For this review, take the finished solid that the model builds, in its own axes (mm). A direction names the side the tool comes from. Give positions to 0.01 mm unless a question says otherwise; leave off trailing zeros. Write each loop counter-clockwise with the first axis right and the second up, starting at its lowest first coordinate (ties: lowest second). Pieces come first, ordered by that corner, then holes. Notation, with made-up numbers: (17.25, -11) -> (57.25, -11) arc R11 ccw to (57.25, 2) -> close; hole circle Ø11 at (85, 15). An arc over 180 degrees is marked (long way). Return JSON: item names as keys, results as strings.
Autodesk Inventor part; units mm, degrees
ref_plane "YZ Plane" through (0, 0, 0) normal (1, 0, 0) x (0, 1, 0)
ref_plane "XZ Plane" through (0, 0, 0) normal (0, 1, 0) x (-1, 0, 0)
ref_plane "XY Plane" through (0, 0, 0) normal (0, 0, 1) x (1, 0, 0)
sketch "Sketch1" plane through (0, 0, 0) normal (0, 0, 1) x (1, 0, 0)
  line L0 (0, 0) -> (92, 0)
  line L1 (92, 0) -> (92, 87.5)
  line L2 (0, 87.5) -> (0, 0)
  line L3 (0, 87.5) -> (4, 91.5)
  line L4 (92, 87.5) -> (88, 91.5)
  line L5 (4, 91.5) -> (4, 183.5)
  line L6 (88, 91.5) -> (88, 151.5)
  line L7 (34.5, 21) -> (57.5, 21)
  line L8 (58.5, 20) -> (58.5, 11)
  line L9 (57.5, 10) -> (34.5, 10)
  line L10 (33.5, 11) -> (33.5, 20)
  arc A0 (34.5, 21) -> (33.5, 20) centre (34.5, 20) ccw
  arc A1 (33.5, 11) -> (34.5, 10) centre (34.5, 11) ccw
  arc A2 (57.5, 10) -> (58.5, 11) centre (57.5, 11) ccw
  arc A3 (58.5, 20) -> (57.5, 21) centre (57.5, 20) ccw
  line L11 (9, 75) -> (32, 75)
  line L12 (33, 74) -> (33, 65)
  line L13 (32, 64) -> (9, 64)
  line L14 (8, 65) -> (8, 74)
  arc A4 (9, 75) -> (8, 74) centre (9, 74) ccw
  arc A5 (8, 65) -> (9, 64) centre (9, 65) ccw
  arc A6 (32, 64) -> (33, 65) centre (32, 65) ccw
  arc A7 (33, 74) -> (32, 75) centre (32, 74) ccw
  arc A8 (59, 65) -> (60, 64) centre (60, 65) ccw
  arc A9 (60, 75) -> (59, 74) centre (60, 74) ccw
  line L15 (83, 64) -> (60, 64)
  line L16 (84, 74) -> (84, 65)
  arc A10 (83, 64) -> (84, 65) centre (83, 65) ccw
  arc A11 (84, 74) -> (83, 75) centre (83, 74) ccw
  line L17 (60, 75) -> (83, 75)
  line L18 (59, 65) -> (59, 74)
  line L19 (4, 183.5) -> (36, 183.5)
  line L20 (36, 183.5) -> (36, 151.5)
  line L21 (36, 151.5) -> (88, 151.5)
  point P0 (46, 10)
  point P1 (46, 0)
  point P2 (84, 69.5)
  point P3 (58.5, 15.5)
  dimension "d0" = 92
  dimension "d1" = 135
  dimension "d2" = 1
  dimension "d3" = 11
  dimension "d4" = 25
  dimension "d5" = 1
  dimension "d6" = 11
  dimension "d7" = 25
  dimension "d8" = 1
  dimension "d9" = 11
  dimension "d10" = 25
  dimension "d11" = 4
  dimension "d12" = 54
  dimension "d13" = 8
  dimension "d14" = 8
  dimension "d15" = 10
  dimension "d16" = 32
  dimension "d17" = 32
  dimension "d18" = 183.5
  dimension "d19" = 87.5
extrude "Extrusion1" add sketch "Sketch1" along normal blind 6
sketch "Sketch2" plane through (0, 0, 6) normal (0, 0, 1) x (1, 0, 0)
  line L0 (34.5, 21) -> (57.5, 21)
  line L1 (33.5, 11) -> (33.5, 20)
  line L2 (34, 23) -> (58, 23) construction
  line L3 (58, 23) -> (58, 8) construction
  line L4 (58, 8) -> (34, 8) construction
  line L5 (34, 8) -> (34, 23) construction
  circle A0 centre (31.75, 32) radius 2.25
  circle A1 centre (60.25, 32) radius 2.25
  line L6 (31.75, 32) -> (60.25, 32) construction
  point P0 (34, 15.5)
  point P1 (33.5, 15.5)
  point P2 (46, 23)
  point P3 (46, 21)
  point P4 (46, 32)
  dimension "d22" = 24
  dimension "d23" = 15
  dimension "d24" = 4.5
  dimension "d25" = 28.5
  dimension "d26" = 9
extrude "Extrusion2" cut sketch "Sketch2" against normal blind 6
sketch "Sketch3" plane through (0, 0, 6) normal (0, 0, 1) x (1, 0, 0)
  circle A0 centre (31.75, 32) radius 2.25
  circle A1 centre (60.25, 32) radius 2.25
  line L0 (16.25, 35) -> (24.25, 35)
  line L1 (24.25, 35) -> (24.25, 29)
  line L2 (24.25, 29) -> (16.25, 29)
  line L3 (16.25, 29) -> (16.25, 35)
  line L4 (67.75, 35) -> (75.75, 35)
  line L5 (75.75, 35) -> (75.75, 29)
  line L6 (75.75, 29) -> (67.75, 29)
  line L7 (67.75, 29) -> (67.75, 35)
  point P0 (24.25, 32)
  dimension "d29" = 6
  dimension "d30" = 8
  dimension "d31" = 8
  dimension "d32" = 7.5
  dimension "d33" = 7.5
extrude "Extrusion3" cut sketch "Sketch3" against normal blind 6 contours L0 L1 L2 L3 | L4 L5 L6 L7
equation "\"d14\" = d13"
properties part number "x_carriage_front"
1. Add section D-D, the plane y = 157.5. State the section outline as (x, z) points, plus the area to 3 significant figures.
Results found:
{"outline": "(4, 0) -> (36, 0) -> (36, 6) -> (4, 6) -> close", "area": "192 mm²"}
2. The part is to be moulded in two halves that separate along X. For faces 1 (the flat face through (88, 121, 3)), 2 (the flat face through (62, 151.5, 3)), 3 (the flat face through (46, 10, 3)), say which applies: +X half, -X half, draft (parallel to the pull), parting line (faces both ways), or undercut.
Results found:
{"face 1": "+X half", "face 2": "draft", "face 3": "undercut"}
3. To check wall thickness, follow probe 1 along Y at (x, z) = (31.75, 4.55); probe 2 along Y at (x, z) = (60.25, 2.5); probe 3 along X at (y, z) = (68.5, 0.45). State the ranges of each line that lie inside material, in increasing order.
Results found:
{"probe 1": "y = 0 to 29.75, 34.25 to 64, 75 to 183.5", "probe 2": "y = 0 to 29.75, 34.25 to 64, 75 to 151.5", "probe 3": "x = 0 to 8, 33 to 59, 84 to 92"}
4. Add section B-B, the plane x = 47.5. State the section outline as (y, z) points, plus the area to 3 significant figures.
Results found:
{"outline": "(0, 0) -> (10, 0) -> (10, 6) -> (0, 6) -> close; (21, 0) -> (151.5, 0) -> (151.5, 6) -> (21, 6) -> close", "area": "843 mm²"}
5. For faces 4 (the flat face through (20, 75, 3)), 5 (the flat face through (45, 93, 0)), list the 3-axis set-ups (+Z, -Z, +X, -X, +Y, -Y) from which the entire face can be reached by the end or side of a thin tool; tool diameter is ignored.
Results found:
{"face 4": "+Z, -Z", "face 5": "-Z, +X, -X, +Y, -Y"}
6. For pin 1 (1.8 mm diameter, centred on y = 172.5, z = 1.5, fed in from +X); pin 2 (1.8 mm diameter, centred on y = 154, z = 3.5, fed in from -X), all flat-tipped, find the tip position at first contact; note any pin that passes through.
Results found:
{"pin 1": "stops at x = 36", "pin 2": "stops at x = 4"}
7. Add section A-A, the plane y = 32. State the section outline as (x, z) points.
Results found:
{"outline": "(0, 0) -> (16.25, 0) -> (16.25, 6) -> (0, 6) -> close; (24.25, 0) -> (29.5, 0) -> (29.5, 6) -> (24.25, 6) -> close; (34, 0) -> (58, 0) -> (58, 6) -> (34, 6) -> close; (62.5, 0) -> (67.75, 0) -> (67.75, 6) -> (62.5, 6) -> close; (75.75, 0) -> (92, 0) -> (92, 6) -> (75.75, 6) -> close"}
8. Add section C-C, the plane z = 2.2. Count the separate pieces of the cut face and the enclosed holes in it, plus the area to 3 significant figures.
Results found:
{"separate pieces": "1", "enclosed holes": "7", "area": "13,500 mm²"}
